Read the model definition and answer for the solid it produces. Units are mm, in the model's axes. A direction names the side the tool comes from. Give positions to 0.01 mm unless a question says otherwise; leave off trailing zeros. Write each loop counter-clockwise with the first axis right and the second up, starting at its lowest first coordinate (ties: lowest second). Pieces come first, ordered by that corner, then holes. Notation, with made-up numbers: (1, 73.5) -> (29, 73.5) arc R21 ccw to (29, 100.5) -> close; hole circle Ø9 at (18, 26.5). An arc over 180 degrees is marked (long way). Use a Markdown table: item, result.
from build123d import *

# Parameters (mm, degrees)
BOSS_EXTRUDE1_DEPTH = 2350


with BuildPart() as part:
    # Sketch1 → Boss-Extrude1 (new body)
    with BuildSketch(Plane(origin=(0, 2350, 0), x_dir=(1, 0, 0), z_dir=(0, 1, 0))):
        with BuildLine():
            Line((25, 75), (49, 75))
            Line((49, 75), (49, 50))
            Line((49, 50), (89, 50))
            Line((89, 50), (89, 0))
            Line((89, 0), (59, 0))
            Line((59, 0), (59, -6))
            Line((59, -6), (95, -6))
            Line((95, -6), (95, 56))
            Line((95, 56), (55, 56))
            Line((55, 56), (55, 81))
            Line((55, 81), (21.540600907, 81))
            ThreePointArc((21.540600907, 81), (0, 67.583123952), (-21.540600907, 81))
            Line((-21.540600907, 81), (-55, 81))
            Line((-55, 81), (-55, 56))
            Line((-55, 56), (-95, 56))
            Line((-95, 56), (-95, -6))
            Line((-95, -6), (-59, -6))
            Line((-59, -6), (-59, 0))
            Line((-59, 0), (-89, 0))
            Line((-89, 0), (-89, 50))
            Line((-89, 50), (-49, 50))
            Line((-49, 50), (-49, 75))
            Line((-49, 75), (-25, 75))
            ThreePointArc((-25, 75), (0, 61.583123952), (25, 75))
        make_face()
    extrude(amount=-BOSS_EXTRUDE1_DEPTH)


solid = part.part
Item 1: Straight lines are drawn through the part: line 1 along X through (y, z) = (1626, -4); line 2 along X through (y, z) = (1186.5, -52.5); line 3 along Z through (x, y) = (83.5, 1584.5). For each, find the intervals that lie inside material, in ascending order. Write a range as [from, to].
Return value:
| item | result |
|---|---|
| line 1 | [-95, -89], [89, 95] |
| line 2 | [-95, -49], [49, 95] |
| line 3 | [-56, -50], [0, 6] |
Item 2: A cutting plane is placed at A-A (z = -24). Give the vertices of the cut face in (x, y).
Return value:
| item | result |
|---|---|
| outline | (-95, 0) -> (-89, 0) -> (-89, 2350) -> (-95, 2350) -> close; (89, 0) -> (95, 0) -> (95, 2350) -> (89, 2350) -> close |
Item 3: A tool of negligible diameter and unlimited length cuts with its end or side. For faces 1 (the face through (-89, 1191, -25)), 2 (the face through (-75, 1191, -56)), 3 (the face through (75, 1191, -56)), from which of +Z, -Z, +X, -X, +Y, -Y can it reach the whole face along a straight path? Write none if from no direction.
Return value:
| item | result |
|---|---|
| face 1 | +Y, -Y |
| face 2 | -Z, -X, +Y, -Y |
| face 3 | -Z, +X, +Y, -Y |
Item 4: For a pull along X with two mould halves and no side action, classify faces 4 (the face through (-69, 1191, -50)), 5 (the face through (-7, 2350, -63)), 6 (the face through (95, 1191, -25)) as +X half, -X half, draft (parallel to the pull), parting line (faces both ways), or undercut.
Return value:
| item | result |
|---|---|
| face 4 | undercut |
| face 5 | draft |
| face 6 | +X half |
Item 5: Each of these flat-tipped pins is pushed along its axis until it touches: P1, Ø7.5, axis at y = 927.5, z = -68.5, coming from the +X side; P2, Ø2, axis at x = -49, z = -48, coming from the +Y side; P3, Ø24, axis at x = 67.5, y = 1065.5, coming from the -Z side; P4, Ø12.5, axis at y = 746.5, z = -59.5, coming from the -X side. Where does it stop, or does it pass through?
Return value:
| item | result |
|---|---|
| P1 | x = 55 |
| P2 | through |
| P3 | z = -56 |
| P4 | x = -95 |
Item 6: A cutting plane is placed at B-B (y = 1907). Give the vertices of the cut face in (x, z), then the cut area to 3 significant figures.
Return value:
| item | result |
|---|---|
| outline | (-95, -56) -> (-55, -56) -> (-55, -81) -> (-21.54, -81) arc R24 cw to (21.54, -81) -> (55, -81) -> (55, -56) -> (95, -56) -> (95, 6) -> (59, 6) -> (59, 0) -> (89, 0) -> (89, -50) -> (49, -50) -> (49, -75) -> (25, -75) arc R30 ccw to (-25, -75) -> (-49, -75) -> (-49, -50) -> (-89, -50) -> (-89, 0) -> (-59, 0) -> (-59, 6) -> (-95, 6) -> close |
| area | 2,530 mm^2 |
